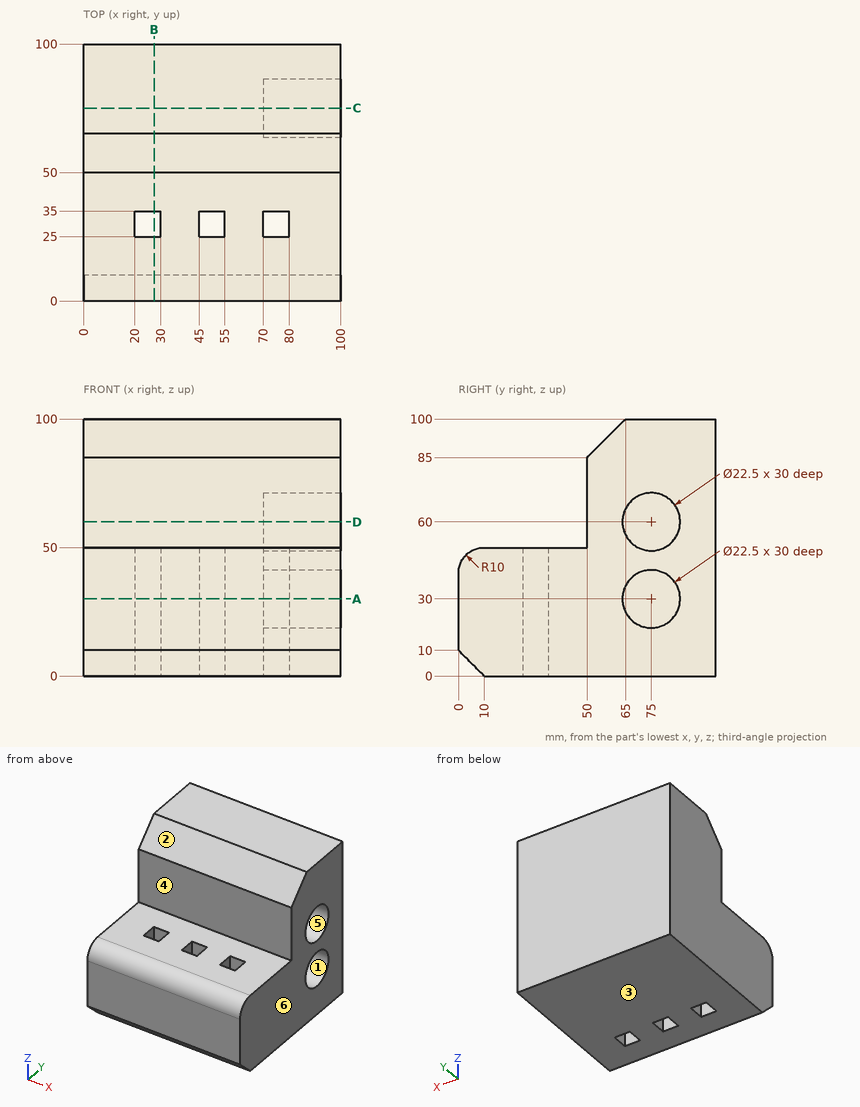
Source: three-view drawing plus pictorial views. Frame: mm from the lowest corner of the part. A direction names the side the tool comes from. Give positions to 0.01 mm unless a question says otherwise; leave off trailing zeros. Write each loop counter-clockwise with the first axis right and the second up, starting at its lowest first coordinate (ties: lowest second). Pieces come first, ordered by that corner, then holes. Notation, with made-up numbers: (-24.75, 62.25) -> (3.25, 62.25) arc R25 cw to (3.25, 98.25) -> close; hole circle Ø3 at (20, -32.5). An arc over 180 degrees is marked (long way). Answer in a Markdown table with one row per item.
(1) Set-up query: the marked faces 4, 5 and 6. Return all of +Z, -Z, +X, -X, +Y, -Y with unobstructed straight access to the full face (end or side cutting, diameter ignored); none if empty.
Answers below:
| item | result |
|---|---|
| face 4 | +Z, +X, -X, -Y |
| face 5 | +X |
| face 6 | +Z, -Z, +X, +Y, -Y |
(2) Section query C-C on y = 75. Return loops of the section in (x, z), then the cut area to 3 significant figures.
Answers below:
| item | result |
|---|---|
| outline | (0, 0) -> (100, 0) -> (100, 18.75) -> (70, 18.75) -> (70, 41.25) -> (100, 41.25) -> (100, 48.75) -> (70, 48.75) -> (70, 71.25) -> (100, 71.25) -> (100, 100) -> (0, 100) -> close |
| area | 8,650 mm^2 |
(3) Section query D-D on z = 60. Return loops of the section in (x, y), then the cut area to 4 significant figures.
Answers below:
| item | result |
|---|---|
| outline | (0, 50) -> (100, 50) -> (100, 63.75) -> (70, 63.75) -> (70, 86.25) -> (100, 86.25) -> (100, 100) -> (0, 100) -> close |
| area | 4,325 mm^2 |
(4) Ray query, line 1 along Z through (x, y) = (77, 75); line 2 along Y through (x, z) = (76, 25.5); line 3 along Z through (x, y) = (75, 16). Return the intervals inside material, ascending. Write a range as [from, to].
Answers below:
| item | result |
|---|---|
| line 1 | [0, 18.75], [41.25, 48.75], [71.25, 100] |
| line 2 | [0, 25], [35, 64.69], [85.31, 100] |
| line 3 | [0, 50] |
(5) Section query A-A on z = 30. Return loops of the section in (x, y).
Answers below:
| item | result |
|---|---|
| outline | (0, 0) -> (100, 0) -> (100, 63.75) -> (70, 63.75) -> (70, 86.25) -> (100, 86.25) -> (100, 100) -> (0, 100) -> close; hole (20, 25) -> (30, 25) -> (30, 35) -> (20, 35) -> close; hole (45, 25) -> (55, 25) -> (55, 35) -> (45, 35) -> close; hole (70, 25) -> (80, 25) -> (80, 35) -> (70, 35) -> close |
(6) Pin query (flat end, axial travel): pin 1 (3 mm diameter, centred on x = 76, y = 45, fed in from +Z); pin 2 (18 mm diameter, centred on y = 75, z = 60, fed in from +X). Return the tip coordinate at first contact, or that it passes through.
Answers below:
| item | result |
|---|---|
| pin 1 | z = 50 |
| pin 2 | x = 70 |
(7) Draft query along Z for the marked faces 1, 2 and 3. Return one class per face: +Z half, -Z half, draft (parallel to the pull), parting line (faces both ways), or undercut.
Answers below:
| item | result |
|---|---|
| face 1 | undercut |
| face 2 | +Z half |
| face 3 | -Z half |
(8) Section query B-B on x = 27.5. Return loops of the section in (y, z), then the cut area to 3 significant figures.
Answers below:
| item | result |
|---|---|
| outline | (0, 10) -> (10, 0) -> (25, 0) -> (25, 50) -> (10, 50) arc R10 ccw to (0, 40) -> close; (35, 0) -> (100, 0) -> (100, 100) -> (65, 100) -> (50, 85) -> (50, 50) -> (35, 50) -> close |
| area | 6,820 mm^2 |
